from build123d import *

# Parameters (mm, degrees)
SKETCH1_R           = 5
BOSS_EXTRUDE1_DEPTH = 2
SKETCH4_R           = 3.9
BOSS_EXTRUDE2_DEPTH = 16
SKETCH6_R           = 2.45
SKETCH6_R_2         = 1.6
BOSS_EXTRUDE3_DEPTH = 16


with BuildPart() as part:
    # Sketch1 → Boss-Extrude1 (new body)
    with BuildSketch(Plane(origin=(0, 0, 0), x_dir=(1, 0, 0), z_dir=(0, 1, 0))):
        Circle(SKETCH1_R)
    extrude(amount=BOSS_EXTRUDE1_DEPTH)

    # Sketch4 → Boss-Extrude2 (add)
    with BuildSketch(Plane(origin=(0, 0, 0), x_dir=(-1, 0, 0), z_dir=(0, -1, 0))):
        Circle(SKETCH4_R)
    extrude(amount=BOSS_EXTRUDE2_DEPTH)

    # Sketch6 → Boss-Extrude3 (add)
    with BuildSketch(Plane(origin=(0, -16, 0), x_dir=(-1, 0, 0), z_dir=(0, -1, 0))):
        Circle(SKETCH6_R)
        Circle(SKETCH6_R_2, mode=Mode.SUBTRACT)
    extrude(amount=BOSS_EXTRUDE3_DEPTH)


solid = part.part
The listing builds one solid part. Answer for the finished solid, in the listing's coordinates (mm). A direction names the side the tool comes from. Give positions to 0.01 mm unless a question says otherwise; leave off trailing zeros. Loops run counter-clockwise (first coordinate to the right, second up) from the corner with the lowest first, then second, coordinate; pieces in that order, holes last.
Item 1: A cutting plane is placed at C-C (x = 0). Give the vertices of the cut face in (y, z).
Derived:
outline: (-32, -2.45) - (-16, -2.45) - (-16, -3.9) - (0, -3.9) - (0, -5) - (2, -5) - (2, 5) - (0, 5) - (0, 3.9) - (-16, 3.9) - (-16, 2.45) - (-32, 2.45) - (-32, 1.6) - (-16, 1.6) - (-16, -1.6) - (-32, -1.6) - close
Item 2: A cutting plane is placed at B-B (z = 0). Give the vertices of the cut face in (x, y).
Derived:
outline: (-5, 0) - (-3.9, 0) - (-3.9, -16) - (-2.45, -16) - (-2.45, -32) - (-1.6, -32) - (-1.6, -16) - (1.6, -16) - (1.6, -32) - (2.45, -32) - (2.45, -16) - (3.9, -16) - (3.9, 0) - (5, 0) - (5, 2) - (-5, 2) - close
Item 3: A tool of negligible diameter and unlimited length cuts with its end or side. For faces 1 (the cylindrical face through (-1.08, 0.99, 4.88)), 2 (the cylindrical face through (0.5, -23.9, 2.4)), from which of +Z, -Z, +X, -X, +Y, -Y can it reach the whole face along a straight path? Write none if from no direction.
Derived:
face 1: +Y, -Y
face 2: -Y
Item 4: A cutting plane is placed at A-A (y = -20.5). Give the vertices of the cut face in (x, z), then the cut area to 3 significant figures.
Derived:
outline: circle Ø4.9 at (0, 0); hole circle Ø3.2 at (0, 0)
area: 10.8 mm2
Item 5: Find the intervals of material crossed by line 1 along X through (y, z) = (-27, 0); line 2 along Y through (x, z) = (-2.25, -3.25), in increasing order.
Derived:
line 1: x = -2.45 to -1.6, 1.6 to 2.45
line 2: y = 0 to 2
Item 6: Each of these flat-tipped pins is pushed along its axis until it touches: pin 1 Ø2.5 at (x, z) = (0, 0) entering from -Y; pin 2 Ø2 at (y, z) = (-19.5, -3) entering from -X; pin 3 Ø4 at (y, z) = (-21, 3) entering from -X. Where does it stop, or does it pass through?
Derived:
pin 1: stops at y = -16
pin 2: stops at x = -1.42
pin 3: stops at x = -2.24
Item 7: A cutting plane is placed at D-D (y = -1.5). Give the vertices of the cut face in (x, z).
Derived:
outline: circle Ø7.8 at (0, 0)
